Source: CAD feature listing. Evaluate the final solid. Frame: model axes, mm. Face numbers are marked on the shaded views. Round coordinates to 2 decimals unless told otherwise and drop trailing zeros. Write each loop counter-clockwise with the first axis right and the second up, starting at its lowest first coordinate (ties: lowest second). Pieces come first, ordered by that corner, then holes. Notation, with made-up numbers: (47.5, -36) -> (54.5, -36) arc R22 cw to (54.5, -17) -> close; hole circle Ø4 at (22, 42.5). An arc over 180 degrees is marked (long way). Put each result on its own line as item: value.
```python
from build123d import *

# Parameters (mm, degrees)
SKETCH_1_R           = 2.1
EXTRUDE_2_DEPTH      = 8
SKETCH_2_R           = 2.2
CUT_EXTRUDE_1_DEPTH  = 20
SKETCH_2_3_R         = 4
SKETCH_2_3_R_2       = 2.2
CUT_EXTRUDE_2_DEPTH  = 2
CUT_EXTRUDE_START    = -8
SKETCH_9_R           = 3
SKETCH_9_R_2         = 2.1
CUT_EXTRUDE_11_DEPTH = 8
SKETCH_10_R          = 5.6
SKETCH_10_R_2        = 3
CUT_EXTRUDE_12_DEPTH = 5.5
SKETCH_10_3_R        = 6
SKETCH_10_3_R_2      = 5.6
CUT_EXTRUDE_13_DEPTH = 5.5
SKETCH_10_4_R        = 5.6
SKETCH_10_4_R_2      = 3
CUT_EXTRUDE_14_DEPTH = 20
CHAMFER_1_SIZE       = 0.2
SKETCH_11_R          = 2.2
EXTRUDE_3_DEPTH      = 8
FILLET_1_R           = 5
SKETCH_12_W          = 11
SKETCH_12_H          = 3
EXTRUDE_5_DEPTH      = 2
CUT_EXTRUDE_START_2  = -2
SKETCH_13_R          = 4
CUT_EXTRUDE_16_DEPTH = 2
CHAMFER_2_SIZE       = 0.2


with BuildPart() as part:
    # 스케치1 → 보스-돌출2 (new body)
    with BuildSketch(Plane(origin=(0, 0, 0), x_dir=(1, 0, 0), z_dir=(0, 1, 0))):
        with BuildLine():
            Line((34.25, 8.714212529), (4.25, 16.460179221))
            ThreePointArc((4.25, 16.460179221), (-17, 0), (4.25, -16.460179221))
            Line((4.25, -16.460179221), (34.25, -8.714212529))
            ThreePointArc((34.25, -8.714212529), (41, 0), (34.25, 8.714212529))
        make_face()
        with Locations(Location((32, 0, 0), (0, 0, 270))):
            Circle(SKETCH_1_R, mode=Mode.SUBTRACT)
    extrude(amount=EXTRUDE_2_DEPTH)

    # 스케치2 → 컷-돌출1 (cut)
    with BuildSketch(Plane(origin=(0, 8, 0), x_dir=(1, 0, 0), z_dir=(0, 1, 0))):
        with Locations(Location((0, 0, 0), (0, 0, 270))):
            Circle(SKETCH_2_R)
    extrude(amount=-CUT_EXTRUDE_1_DEPTH, mode=Mode.SUBTRACT)

    # 스케치2<3> → 컷-돌출2 (cut)
    with BuildSketch(Plane(origin=(0, 8, 0), x_dir=(1, 0, 0), z_dir=(0, 1, 0))):
        with Locations(Location((0, 0, 0), (0, 0, 270))):
            Circle(SKETCH_2_3_R)
        with Locations(Location((0, 0, 0), (0, 0, 270))):
            Circle(SKETCH_2_3_R_2, mode=Mode.SUBTRACT)
    extrude(amount=-CUT_EXTRUDE_2_DEPTH, mode=Mode.SUBTRACT)

    # 스케치9 → 컷-돌출11 (cut)
    with BuildSketch(Plane(origin=(0, 8, 0), x_dir=(1, 0, 0), z_dir=(0, 1, 0)).offset(CUT_EXTRUDE_START)):
        with Locations(Location((32, 0, 0), (0, 0, 270))):
            Circle(SKETCH_9_R)
        with Locations((32, 0)):
            Circle(SKETCH_9_R_2, mode=Mode.SUBTRACT)
    extrude(amount=CUT_EXTRUDE_11_DEPTH, mode=Mode.SUBTRACT)

    # 스케치10 → 컷-돌출12 (cut)
    with BuildSketch(Plane.XZ):
        with Locations(Location((32, 0, 0), (0, 0, 270))):
            Circle(SKETCH_10_R)
        with Locations(Location((32, 0, 0), (0, 0, 90))):
            Circle(SKETCH_10_R_2, mode=Mode.SUBTRACT)
    extrude(amount=-CUT_EXTRUDE_12_DEPTH, mode=Mode.SUBTRACT)

    # 스케치10<3> → 컷-돌출13 (cut)
    with BuildSketch(Plane.XZ):
        with Locations(Location((32, 0, 0), (0, 0, 270))):
            Circle(SKETCH_10_3_R)
        with Locations((32, 0)):
            Circle(SKETCH_10_3_R_2, mode=Mode.SUBTRACT)
    extrude(amount=-CUT_EXTRUDE_13_DEPTH, mode=Mode.SUBTRACT)

    # 스케치10<4> → 컷-돌출14 (cut)
    with BuildSketch(Plane.XZ):
        with Locations(Location((32, 0, 0), (0, 0, 270))):
            Circle(SKETCH_10_4_R)
        with Locations((32, 0)):
            Circle(SKETCH_10_4_R_2, mode=Mode.SUBTRACT)
    extrude(amount=-CUT_EXTRUDE_14_DEPTH, mode=Mode.SUBTRACT)

    # 모따기1
    chamfer_1_edges = [part.edges().sort_by_distance(p)[0] for p in [
        (32, 0, 6),
        (32, 8, 5.6),
    ]]
    chamfer(chamfer_1_edges, length=CHAMFER_1_SIZE)

    # 스케치11 → 보스-돌출3 (add)
    # profile 1 of 3: a face of its own
    with BuildSketch(Plane(origin=(0, 0, 0), x_dir=(1, 0, 0), z_dir=(0, 1, 0))):
        with BuildLine():
            ThreePointArc((-17, 1.7e-08), (-13.43968005, 10.410331414), (-4.25, 16.460179221))
            Line((-4.25, 16.460179221), (-17, 13.168143377))
            Line((-17, 13.168143377), (-17, 1.7e-08))
        make_face()
    # profile 2 of 3: a face of its own
    with BuildSketch(Plane(origin=(0, 0, 0), x_dir=(1, 0, 0), z_dir=(0, 1, 0))):
        with BuildLine():
            ThreePointArc((-4.25, -16.460179221), (-13.439680061, -10.4103314), (-17, 1.7e-08))
            Line((-17, 1.7e-08), (-17, -13.168143377))
            Line((-17, -13.168143377), (-4.25, -16.460179221))
        make_face()
    # profile 3 of 3: a face of its own
    with BuildSketch(Plane(origin=(0, 0, 0), x_dir=(1, 0, 0), z_dir=(0, 1, 0))):
        Polygon((-17, 1.7e-08), (-17, 13.168143377), (-28, 10.32795559), (-28, -10.32795559), (-17, -13.168143377), align=None)
        with Locations(Location((-22.5, -6, 0), (0, 0, 270))):
            Circle(SKETCH_11_R, mode=Mode.SUBTRACT)
        with Locations(Location((-22.5, 6, 0), (0, 0, 270))):
            Circle(SKETCH_11_R, mode=Mode.SUBTRACT)
    extrude(amount=EXTRUDE_3_DEPTH)

    # 필렛1
    fillet_1_edges = [part.edges().sort_by_distance(p)[0] for p in [
        (-28, 4, 10.32795559),
        (-28, 4, -10.32795559),
    ]]
    fillet(fillet_1_edges, radius=FILLET_1_R)

    # 스케치12 → 보스-돌출5 (add)
    with BuildSketch(Plane(origin=(0, 8, 0), x_dir=(1, 0, 0), z_dir=(0, 1, 0))):
        with Locations((-22.5, 0)):
            Rectangle(SKETCH_12_W, SKETCH_12_H)
    extrude(amount=EXTRUDE_5_DEPTH)

    # 스케치13 → 컷-돌출16 (cut)
    with BuildSketch(Plane.XZ.offset(CUT_EXTRUDE_START_2)):
        with Locations(Location((-22.5, 6, 0), (0, 0, 270))):
            Circle(SKETCH_13_R)
        with Locations(Location((-22.5, -6, 0), (0, 0, 270))):
            Circle(SKETCH_13_R)
        with Locations(Location((0, 0, 0), (0, 0, 90))):
            Circle(SKETCH_13_R)
    extrude(amount=CUT_EXTRUDE_16_DEPTH, mode=Mode.SUBTRACT)

    # 모따기2
    chamfer_2_edges = [part.edges().sort_by_distance(p)[0] for p in [
        (-28, 8, -3.977486122),
        (-26.952847075, 8, -9.516834422),
        (-26.952847075, 8, 9.516834422),
        (19.25, 8, -12.587195875),
        (-28, 8, 3.977486122),
        (-17, 9, 1.5),
        (-17, 9, -1.5),
        (-28, 9, -1.5),
        (-28, 9, 1.5),
        (-17, 10, 0),
        (-22.5, 10, -1.5),
        (-28, 10, 0),
        (-22.5, 10, 1.5),
        (0, 0, -4),
        (0, 2, -2.2),
        (-22.5, 2, -8.2),
        (-22.5, 0, -2),
        (-22.5, 2, 3.8),
        (-22.5, 0, 10),
        (0, 8, -17),
        (19.25, 8, 12.587195875),
        (0, 6, -2.2),
        (0, 8, -4),
        (41, 8, 0),
        (19.25, 0, 12.587195875),
        (0, 0, -17),
        (0, 0, 17),
        (0, 8, 17),
        (-22.5, 8, 3.8),
        (-14.25, 0, -13.878190324),
        (19.25, 0, -12.587195875),
        (-22.5, 8, -8.2),
        (-14.25, 8, -13.878190324),
        (41, 0, 0),
        (-14.25, 8, 13.878190324),
        (-14.25, 0, 13.878190324),
        (-28, 0, 0),
        (-26.952847075, 0, -9.516834422),
        (-26.952847075, 0, 9.516834422),
    ]]
    chamfer(chamfer_2_edges, length=CHAMFER_2_SIZE)


solid = part.part
```
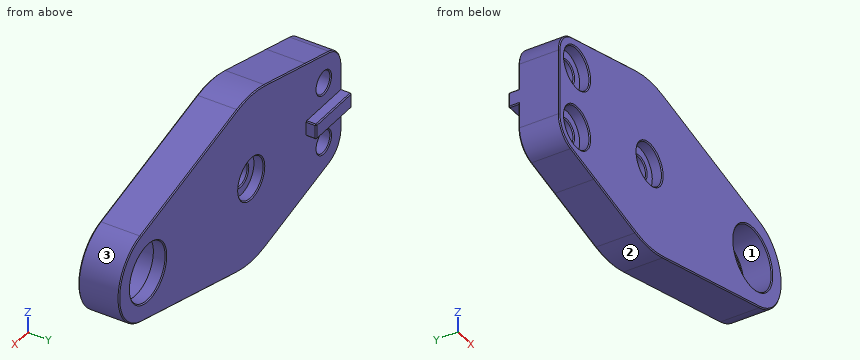
Q1. Cut plane C-C on x = 32. Output: boundary loops of the cut face in (y, z), and give its area (3 significant figures).
Ans:
outline: (0, -9.09) -> (0.2, -9.3) -> (7.8, -9.3) -> (8, -9.09) -> (8, -5.8) -> (7.8, -5.6) -> (5.5, -5.6) -> (5.5, -6) -> (0.2, -6) -> (0, -6.2) -> close; (0, 6.2) -> (0.2, 6) -> (5.5, 6) -> (5.5, 5.6) -> (7.8, 5.6) -> (8, 5.8) -> (8, 9.09) -> (7.8, 9.3) -> (0.2, 9.3) -> (0, 9.09) -> close
area: 54.6 mm^2
Q2. Material intervals for line 1 (X direction, y = 1.45, z = 0); line 2 (X direction, y = 3.1, z = 0); line 3 (Y direction, x = -20.5, z = -3), sorted ascending. Write a range as [from, to].
Ans:
line 1: x = [-28, -4], [4, 26], [38, 41]
line 2: x = [-28, -2.2], [2.2, 26], [38, 41]
line 3: y = [2, 8]
Q3. Cut plane B-B on z = 0. Give the number of separate pieces and of enclosed holes in the cut face, and give its area (3 significant figures).
Ans:
separate pieces: 3
enclosed holes: 0
area: 430 mm^2
Q4. Cut plane D-D on x = 20.5. Output: boundary loops of the cut face in (y, z), and give its area (3 significant figures).
Ans:
outline: (0, -12.06) -> (0.2, -12.26) -> (7.8, -12.26) -> (8, -12.06) -> (8, 12.06) -> (7.8, 12.26) -> (0.2, 12.26) -> (0, 12.06) -> close
area: 196 mm^2
Q5. Draft query along X for the marked faces 1, 2 and 3. Return one class per face: +X half, -X half, draft (parallel to the pull), parting line (faces both ways), or undercut.
Ans:
face 1: undercut
face 2: parting line
face 3: +X half
Q6. Cut plane A-A on y = 1. Output: boundary loops of the cut face in (x, z).
Ans:
outline: (-28, -6.45) arc R5 ccw to (-24.25, -11.3) -> (-4.25, -16.46) arc R17 ccw to (4.25, -16.46) -> (34.25, -8.71) arc R9 ccw to (34.25, 8.71) -> (4.25, 16.46) arc R17 ccw to (-4.25, 16.46) -> (-24.25, 11.3) arc R5 ccw to (-28, 6.45) -> close; hole circle Ø8 at (-22.5, -6); hole circle Ø8 at (-22.5, 6); hole circle Ø8 at (0, 0); hole circle Ø12 at (32, 0)
Q7. Pin query (flat end, axial travel): pin 1 (0.9 mm diameter, centred on x = -24.5, y = 8.5, fed in from +Z); pin 2 (9 mm diameter, centred on x = 1.5, z = -1.5, fed in from +Y); pin 3 (1 mm diameter, centred on x = -15.5, y = 6, fed in from +Z). Return the tip coordinate at first contact, or that it passes through.
Ans:
pin 1: stops at z = 1.5
pin 2: stops at y = 8
pin 3: stops at z = 13.68
